Work out the finished part from the listing and answer in its coordinate system (mm). Round coordinates to 2 decimals unless told otherwise and drop trailing zeros. Order: outer loops, then holes, each group sorted by start corner. A loop starts at its lowest first (then second) coordinate and runs counter-clockwise, first axis right, second up. Notation, with made-up numbers: (62.5, 89) - (75.5, 89) arc R3 ccw to (75.5, 93) - close; hole circle Ø8 at (5.25, 3). An arc over 180 degrees is marked (long way). Use CSV: the item, a comma, the result in double quotes.
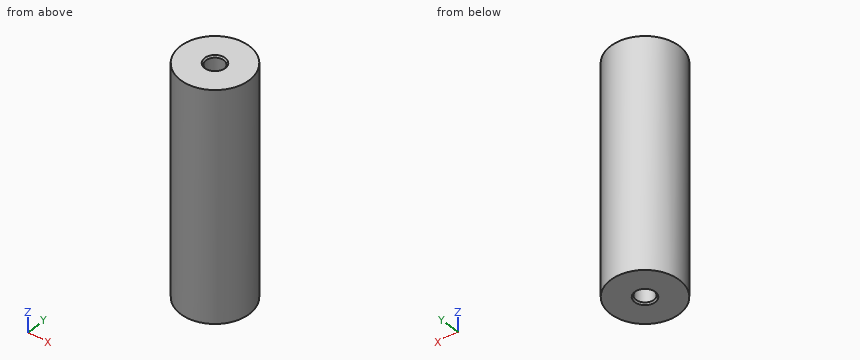
Autodesk Inventor part; units mm, degrees
ref_plane "YZ Plane" through (0, 0, 0) normal (1, 0, 0) x (0, 1, 0)
ref_plane "XZ Plane" through (0, 0, 0) normal (0, 1, 0) x (-1, 0, 0)
ref_plane "XY Plane" through (0, 0, 0) normal (0, 0, 1) x (1, 0, 0)
sketch "Эскиз1" plane through (0, 0, 0) normal (0, 0, 1) x (1, 0, 0)
  circle A0 centre (0, 0) radius 7.5
  dimension "d0" = 15
extrude "Выдавливание1" add sketch "Эскиз1" along normal mid plane 50
sketch "Эскиз2" plane through (0, 0, 25) normal (0, 0, 1) x (1, 0, 0)
  point P0 (0, 0)
hole "Отверстие1" at (0, 0, 25) direction (0, 0, -1) diameter 3.9 depth 10 countersink diameter 4.5 countersink angle 82
mirror "Зеркальное отражение1" about plane through (0, 0, 0) normal (0, 0, 1) of "Отверстие1"
properties part number "Стойка" material "По умолчанию1"
(1) Find section D-D (x = 4.5). Determine the outline of the cut face in (y, z).
Findings below:
outline,"(-6, -25) - (6, -25) - (6, 25) - (-6, 25) - close"
(2) Find the intervals of material crossed by L1, parallel to Y at x = 0, z = -19.25; L2, parallel to Z at x = 1.5, y = 0.5; L3, parallel to X at y = 0.5, z = -12, in increasing order. Write a range as from..to.
Findings below:
L1,"y = -7.5..-1.95, 1.95..7.5"
L2,"z = -15..15"
L3,"x = -7.48..7.48"
(3) Each of these flat-tipped pins is pushed along its axis until it touches: pin 1 (3 mm diameter, centred on x = 0, y = 0, fed in from -Z); pin 2 (5 mm diameter, centred on x = 3.5, z = -1.5, fed in from +Y); pin 3 (3.5 mm diameter, centred on x = 0, y = 0, fed in from +Z). Where does it stop, or does it pass through?
Findings below:
pin 1,"stops at z = -15"
pin 2,"stops at y = 7.43"
pin 3,"stops at z = 15"
(4) Find section A-A (x = 0). Determine the outline of the cut face in (y, z).
Findings below:
outline,"(-7.5, -25) - (-2.25, -25) - (-1.95, -24.65) - (-1.95, -15) - (1.95, -15) - (1.95, -24.65) - (2.25, -25) - (7.5, -25) - (7.5, 25) - (2.25, 25) - (1.95, 24.65) - (1.95, 15) - (-1.95, 15) - (-1.95, 24.65) - (-2.25, 25) - (-7.5, 25) - close"
(5) Find section C-C (z = 11). Determine the outline of the cut face in (x, y), and give its area (3 significant figures).
Findings below:
outline,"circle Ø15 at (0, 0)"
area,"177 mm²"
